from build123d import *

# Parameters (mm, degrees)
SKETCH2_W           = 140
SKETCH2_H           = 60
SKETCH2_R           = 2.1
BOSS_EXTRUDE1_DEPTH = 2.5
SKETCH3_W           = 6
SKETCH3_H           = 8
SKETCH3_W_2         = 10
SKETCH3_H_2         = 30
BOSS_EXTRUDE2_DEPTH = 3.5
SKETCH4_W           = 30
SKETCH4_H           = 20
BOSS_EXTRUDE3_DEPTH = 12.5


with BuildPart() as part:
    # Sketch2 → Boss-Extrude1 (new body)
    with BuildSketch(Plane(origin=(0, 0, 0), x_dir=(1, 0, 0), z_dir=(0, 1, 0))):
        Rectangle(SKETCH2_W, SKETCH2_H)
        with Locations((-65, 25)):
            Circle(SKETCH2_R, mode=Mode.SUBTRACT)
        with Locations((8.25, 25)):
            Circle(SKETCH2_R, mode=Mode.SUBTRACT)
        with Locations((65, 25)):
            Circle(SKETCH2_R, mode=Mode.SUBTRACT)
        with Locations((-65, -25)):
            Circle(SKETCH2_R, mode=Mode.SUBTRACT)
        with Locations((8.25, -25)):
            Circle(SKETCH2_R, mode=Mode.SUBTRACT)
        with Locations((65, -25)):
            Circle(SKETCH2_R, mode=Mode.SUBTRACT)
    extrude(amount=BOSS_EXTRUDE1_DEPTH)

    # Sketch3 → Boss-Extrude2 (add)
    with BuildSketch(Plane(origin=(0, 2.5, 0), x_dir=(1, 0, 0), z_dir=(0, 1, 0))):
        with Locations((-42, 25)):
            Rectangle(SKETCH3_W, SKETCH3_H)
        with Locations((-34, 25)):
            Rectangle(SKETCH3_W, SKETCH3_H)
        with Locations((66.5, 0)):
            Rectangle(SKETCH3_W_2, SKETCH3_H_2)
    extrude(amount=BOSS_EXTRUDE2_DEPTH)

    # Sketch4 → Boss-Extrude3 (add)
    with BuildSketch(Plane(origin=(0, 2.5, 0), x_dir=(1, 0, 0), z_dir=(0, 1, 0))):
        with Locations((27.5, 10)):
            Rectangle(SKETCH4_W, SKETCH4_H)
    extrude(amount=BOSS_EXTRUDE3_DEPTH)


solid = part.part
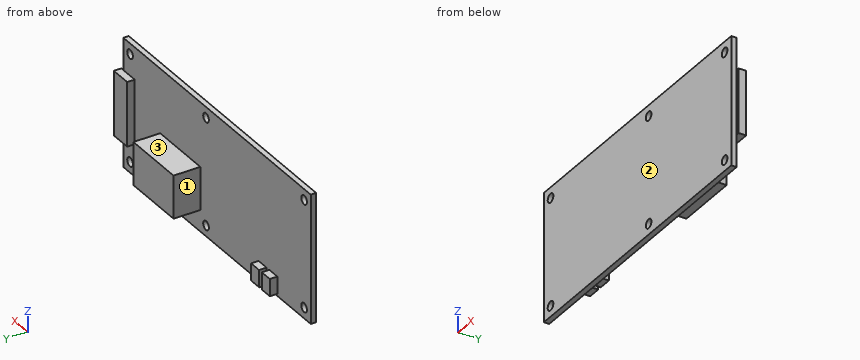
Geometry: final body of the model. Coordinates: model frame, mm. Face numbers are marked on the shaded views. A direction names the side the tool comes from. Coordinates: 2 decimals unless noted, no trailing zeros. Order: outer loops, then holes, each group sorted by start corner. A loop starts at its lowest first (then second) coordinate and runs counter-clockwise, first axis right, second up.
(1) Material intervals for probe 1 along Z at (x, y) = (-65, 1.55); probe 2 along X at (y, z) = (4, -1); probe 3 along X at (y, z) = (9.25, -12.5), sorted ascending.
(2) Section query A-A (z = -25). Return the cut outline in (x, y), plus the area to 4 significant figures.
(3) Access query for the marked faces 1, 2 and 3. Directions: +Z, -Z, +X, -X, +Y, -Y. A direction counts if a zero-diameter tool reaches every point of the face in a straight line with its end or side. Return the directions, or none.
(4) Section query D-D (z = -7.5). Return the cut outline in (x, y), plus the area to 3 significant figures.
(5) First-contact query: pin 1 (6 mm diameter, centred on x = 30, y = 10, fed in from -Z); pin 2 (2 mm diameter, centred on x = 10, z = 14, fed in from +Y); pin 3 (8 mm diameter, centred on x = 53.5, z = 4, fed in from -Y); pin 4 (3 mm diameter, centred on x = -34.5, y = 5, fed in from -Z). Flat tips, straight axial feed; report the tip coordinate or a pass-through.
(6) Section query C-C (x = 19). Return the cut outline in (y, z), plus the area to 3 significant figures.
(7) Section query B-B (x = 65). Return the cut outline in (y, z).
Solution:
1. probe 1: z = -30 to -27.1, -22.9 to 22.9, 27.1 to 30
1. probe 2: x = 12.5 to 42.5, 61.5 to 71.5
1. probe 3: x = 12.5 to 42.5
2. outline: (-70, 0) - (-67.1, 0) - (-67.1, 2.5) - (-70, 2.5) - close; (-62.9, 0) - (6.15, 0) - (6.15, 2.5) - (-31, 2.5) - (-31, 6) - (-37, 6) - (-37, 2.5) - (-39, 2.5) - (-39, 6) - (-45, 6) - (-45, 2.5) - (-62.9, 2.5) - close; (10.35, 0) - (62.9, 0) - (62.9, 2.5) - (10.35, 2.5) - close; (67.1, 0) - (70, 0) - (70, 2.5) - (67.1, 2.5) - close
2. area: 360.5 mm2
3. face 1: +Z, -Z, -X, +Y
3. face 2: +Z, -Z, +X, -X, -Y
3. face 3: +Z, -X, +Y
4. outline: (-70, 0) - (70, 0) - (70, 2.5) - (71.5, 2.5) - (71.5, 6) - (61.5, 6) - (61.5, 2.5) - (42.5, 2.5) - (42.5, 15) - (12.5, 15) - (12.5, 2.5) - (-70, 2.5) - close
4. area: 760 mm2
5. pin 1: stops at z = -20
5. pin 2: stops at y = 2.5
5. pin 3: stops at y = 0
5. pin 4: stops at z = -29
6. outline: (0, -30) - (2.5, -30) - (2.5, -20) - (15, -20) - (15, 0) - (2.5, 0) - (2.5, 30) - (0, 30) - close
6. area: 400 mm2
7. outline: (0, -30) - (2.5, -30) - (2.5, -27.1) - (0, -27.1) - close; (0, -22.9) - (2.5, -22.9) - (2.5, -15) - (6, -15) - (6, 15) - (2.5, 15) - (2.5, 22.9) - (0, 22.9) - close; (0, 27.1) - (2.5, 27.1) - (2.5, 30) - (0, 30) - close
